The listing builds one solid part. Answer for the finished solid, in the listing's coordinates (mm). A direction names the side the tool comes from. Round coordinates to 2 decimals unless told otherwise and drop trailing zeros. Write each loop counter-clockwise with the first axis right and the second up, starting at its lowest first coordinate (ties: lowest second). Pieces come first, ordered by that corner, then holes.
Item 1: Find the intervals of material crossed by probe 1 along X at (y, z) = (14.55, 10); probe 2 along Z at (x, y) = (14.5, 7); probe 3 along Y at (x, z) = (18, 0), in increasing order.
Item 2: Find section D-D on z = -10.5. Give the vertices of the cut face in (x, y), then the cut area to 3 significant figures.
Item 3: Each of these flat-tipped pins is pushed along its axis until it touches: pin 1 (3 mm diameter, centred on x = -9.5, z = 11, fed in from +Y); pin 2 (5 mm diameter, centred on x = -1, z = 25, fed in from +Y); pin 3 (5 mm diameter, centred on x = 12.5, y = 17.5, fed in from +Z); pin 4 (12 mm diameter, centred on x = 3.5, y = 31.5, fed in from +Z). Where does it stop, or does it pass through?
Item 4: Find section B-B on y = 48. Give the vertices of the cut face in (x, z).
Item 5: Find section C-C on z = -25. Give the vertices of the cut face in (x, y), then the cut area to 3 significant figures.
Item 6: A tool of negligible diameter and unlimited length cuts with its end or side. For faces 5 (the face through (-4.22, 19.4, -21.43)), 6 (the face through (0, 5, -23)), 7 (the face through (-4.22, 19.4, 21.43)), 8 (the face through (16.5, 2.5, 25)), 9 (the face through (-7.97, 18.52, -12.21)), from which of +Z, -Z, +X, -X, +Y, -Y can it reach the whole face along a straight path? Write none if from no direction.
Item 7: For a pull along Z with two mould halves and no side action, classify faces 1 (the face through (-11.464, 14.535, -9.239)), 2 (the face through (0, 3, -23.5)), 3 (the face through (12, 39, 0)), 4 (the face through (0, 4, -35)) as +Z half, -Z half, draft (parallel to the pull), parting line (faces both ways), or undercut.
Item 8: Find section A-A on x = 3. Give the vertices of the cut face in (y, z), then the cut area to 3 significant figures.
```python
from build123d import *

# Parameters (mm, degrees)
SKETCH1_W           = 40
SKETCH1_H           = 70
BOSS_EXTRUDE1_DEPTH = 20
SKETCH2_W           = 30
SKETCH2_H           = 24
CUT_EXTRUDE1_DEPTH  = 57.789083458
SKETCH3_R           = 1.65
CUT_EXTRUDE2_DEPTH  = 46
SKETCH5_R           = 3
CUT_EXTRUDE3_DEPTH  = 3
SKETCH9_W           = 6
SKETCH9_H           = 30
CUT_EXTRUDE6_DEPTH  = 57.789083458
CUT_EXTRUDE7_DEPTH  = 10
SKETCH14_W          = 8
SKETCH14_H          = 44
BOSS_EXTRUDE3_DEPTH = 53
SKETCH16_R          = 6.65
CUT_EXTRUDE11_DEPTH = 88.051708771
SKETCH17_R          = 7.65
CUT_EXTRUDE12_DEPTH = 2
FILLET2_R           = 5
SKETCH18_R          = 3
CUT_EXTRUDE13_DEPTH = 18
CHAMFER1_SIZE       = 2
SKETCH19_W          = 7
SKETCH19_H          = 12
CUT_EXTRUDE14_DEPTH = 91.29950166
FILLET4_R           = 2


with BuildPart() as part:
    # Sketch1 → Boss-Extrude1 (new body)
    with BuildSketch(Plane(origin=(0, 0, 0), x_dir=(1, 0, 0), z_dir=(0, 1, 0))):
        Rectangle(SKETCH1_W, SKETCH1_H)
    extrude(amount=BOSS_EXTRUDE1_DEPTH)

    # Sketch2 → Cut-Extrude1 (cut, through all)
    with BuildSketch(Plane.ZY.offset(20)):
        Rectangle(SKETCH2_W, SKETCH2_H)
    extrude(amount=-CUT_EXTRUDE1_DEPTH, mode=Mode.SUBTRACT)

    # Sketch3 → Cut-Extrude2 (cut, through all)
    with BuildSketch(Plane(origin=(0, 20, 0), x_dir=(1, 0, 0), z_dir=(0, 1, 0))):
        with Locations(Location((-10, 10, 0), (0, 0, 270))):
            Circle(SKETCH3_R)
        with Locations(Location((10, 10, 0), (0, 0, 270))):
            Circle(SKETCH3_R)
        with Locations(Location((10, -10, 0), (0, 0, 270))):
            Circle(SKETCH3_R)
        with Locations(Location((-10, -10, 0), (0, 0, 270))):
            Circle(SKETCH3_R)
    extrude(amount=-CUT_EXTRUDE2_DEPTH, mode=Mode.SUBTRACT)

    # Sketch5 → Cut-Extrude3 (cut)
    with BuildSketch(Plane(origin=(0, 20, 0), x_dir=(1, 0, 0), z_dir=(0, 1, 0))):
        with Locations(Location((-10, 10, 0), (0, 0, 270))):
            Circle(SKETCH5_R)
        with Locations(Location((10, 10, 0), (0, 0, 270))):
            Circle(SKETCH5_R)
        with Locations(Location((10, -10, 0), (0, 0, 270))):
            Circle(SKETCH5_R)
        with Locations(Location((-10, -10, 0), (0, 0, 270))):
            Circle(SKETCH5_R)
    extrude(amount=-CUT_EXTRUDE3_DEPTH, mode=Mode.SUBTRACT)

    # Sketch9 → Cut-Extrude6 (cut, through all)
    with BuildSketch(Plane(origin=(20, 0, 0), x_dir=(0, 0, -1), z_dir=(1, 0, 0))):
        with Locations((25, 20)):
            Rectangle(SKETCH9_W, SKETCH9_H)
    cut_extrude6 = extrude(amount=-CUT_EXTRUDE6_DEPTH, mode=Mode.SUBTRACT)

    # Sketch10 → Cut-Extrude7 (cut)
    with BuildSketch(Plane(origin=(0, 5, 0), x_dir=(1, 0, 0), z_dir=(0, 1, 0))):
        with BuildLine():
            Line((15, 23.5), (-15, 23.5))
            ThreePointArc((-15, 23.5), (-16.5, 25), (-15, 26.5))
            Line((-15, 26.5), (15, 26.5))
            ThreePointArc((15, 26.5), (16.5, 25), (15, 23.5))
        make_face()
    cut_extrude7 = extrude(amount=-CUT_EXTRUDE7_DEPTH, mode=Mode.SUBTRACT)

    # Mirror2: Cut-Extrude6, Cut-Extrude7 across plane
    add(cut_extrude6.mirror(Plane.XY), mode=Mode.SUBTRACT)
    add(cut_extrude7.mirror(Plane.XY), mode=Mode.SUBTRACT)

    # Sketch14 → Boss-Extrude3 (add)
    with BuildSketch(Plane(origin=(0, 20, 0), x_dir=(1, 0, 0), z_dir=(0, 1, 0))):
        with Locations((16, 0)):
            Rectangle(SKETCH14_W, SKETCH14_H)
    extrude(amount=BOSS_EXTRUDE3_DEPTH)

    # Sketch16 → Cut-Extrude11 (cut, through all)
    with BuildSketch(Plane.ZY.offset(-12)):
        with Locations((0, 48)):
            Circle(SKETCH16_R)
    extrude(amount=-CUT_EXTRUDE11_DEPTH, mode=Mode.SUBTRACT)

    # Sketch17 → Cut-Extrude12 (cut)
    with BuildSketch(Plane.ZY.offset(-12)):
        with Locations((0, 48)):
            Circle(SKETCH17_R)
    extrude(amount=-CUT_EXTRUDE12_DEPTH, mode=Mode.SUBTRACT)

    # Fillet2
    fillet2_edges = [part.edges().sort_by_distance(p)[0] for p in [
        (16, 73, -22),
        (16, 73, 22),
    ]]
    fillet(fillet2_edges, radius=FILLET2_R)

    # Sketch18 → Cut-Extrude13 (cut)
    with BuildSketch(Plane(origin=(0, 38, 0), x_dir=(1, 0, 0), z_dir=(0, 1, 0))):
        with Locations(Location((10, 10, 0), (0, 0, 270))):
            Circle(SKETCH18_R)
        with Locations(Location((10, -10, 0), (0, 0, 270))):
            Circle(SKETCH18_R)
    extrude(amount=-CUT_EXTRUDE13_DEPTH, mode=Mode.SUBTRACT)

    # Chamfer1
    # the kernel refuses this chamfer: 2 mm, written as the material it takes off along each edge
    with BuildSketch(Plane(origin=(12, 38, 17.379433953), x_dir=(-0.02749587661058651, 0.9996219169112968, 0), z_dir=(0, 0, -1))) as chamfer1_piece_1_section:
        Polygon((CHAMFER1_SIZE * 0.999621916911, CHAMFER1_SIZE * 0.0274958766106), (-CHAMFER1_SIZE * 0.0274958766106, CHAMFER1_SIZE * 0.999621916911), (0, 0), align=None)
    chamfer1_piece_1 = extrude(amount=14.758867907, mode=Mode.PRIVATE)
    chamfer1_piece_1 = chamfer1_piece_1 & Plane(origin=(10, 38.83392746, 10), x_dir=(0, 0, 1), z_dir=(0, 1, 0)) * Cylinder(3, 38, mode=Mode.PRIVATE)
    add(chamfer1_piece_1, mode=Mode.SUBTRACT)
    with BuildSketch(Plane(origin=(12, 38, -2.620566047), x_dir=(-0.02749587661058651, 0.9996219169112968, 0), z_dir=(0, 0, -1))) as chamfer1_piece_2_section:
        Polygon((CHAMFER1_SIZE * 0.999621916911, CHAMFER1_SIZE * 0.0274958766106), (-CHAMFER1_SIZE * 0.0274958766106, CHAMFER1_SIZE * 0.999621916911), (0, 0), align=None)
    chamfer1_piece_2 = extrude(amount=14.758867907, mode=Mode.PRIVATE)
    chamfer1_piece_2 = chamfer1_piece_2 & Plane(origin=(10, 38.833927472, -10), x_dir=(0, 0, 1), z_dir=(0, 1, 0)) * Cylinder(3, 38, mode=Mode.PRIVATE)
    add(chamfer1_piece_2, mode=Mode.SUBTRACT)

    # Sketch19 → Cut-Extrude14 (cut, through all)
    with BuildSketch(Plane(origin=(20, 0, 0), x_dir=(0, 0, -1), z_dir=(1, 0, 0))):
        with Locations((-31.5, 14)):
            Rectangle(SKETCH19_W, SKETCH19_H)
    cut_extrude14 = extrude(amount=-CUT_EXTRUDE14_DEPTH, mode=Mode.SUBTRACT)

    # Mirror3: Cut-Extrude14 across plane
    add(cut_extrude14.mirror(Plane.XY), mode=Mode.SUBTRACT)

    # Fillet4
    fillet4_edges = [part.edges().sort_by_distance(p)[0] for p in [
        (-4, 20, 22),
        (-4, 20, -22),
    ]]
    fillet(fillet4_edges, radius=FILLET4_R)


solid = part.part
```
Check values:
1. probe 1: x = -20 to -11.65, -8.35 to 8.35, 11.65 to 20
1. probe 2: z = -35 to -28, -22 to -15, 15 to 22, 28 to 35
1. probe 3: y = 12 to 41.35, 54.65 to 73
2. outline: (-20, 12) - (-11.57, 12) - (-11.57, 17) - (-12.96, 17) - (-12.96, 20) - (-20, 20) - close; (-8.43, 12) - (8.43, 12) - (8.43, 17) - (7.04, 17) - (7.04, 20) - (-7.04, 20) - (-7.04, 17) - (-8.43, 17) - close; (11.57, 12) - (20, 12) - (20, 73) - (12, 73) - (12, 40) - (12.96, 39.04) - (12.96, 17) - (11.57, 17) - close
2. area: 658 mm2
3. pin 1: stops at y = 17
3. pin 2: stops at y = 5
3. pin 3: stops at z = 22
3. pin 4: passes through
4. outline: (12, -22) - (20, -22) - (20, -6.65) - (14, -6.65) - (14, -7.65) - (12, -7.65) - close; (12, 7.65) - (14, 7.65) - (14, 6.65) - (20, 6.65) - (20, 22) - (12, 22) - close
5. outline: (-20, 0) - (-16.5, 0) - (-16.5, 5) - (-20, 5) - close; (16.5, 0) - (20, 0) - (20, 5) - (16.5, 5) - close
5. area: 35.0 mm2
6. face 5: -Z, -X, +Y
6. face 6: +X, -X, +Y
6. face 7: +Z, -X, +Y
6. face 8: +Y, -Y
6. face 9: +Y
7. face 1: undercut
7. face 2: undercut
7. face 3: draft
7. face 4: -Z half
8. outline: (0, -35) - (8, -35) - (8, -28) - (5, -28) - (5, -26.5) - (0, -26.5) - close; (0, -23.5) - (5, -23.5) - (5, -22) - (18, -22) arc R2 ccw to (20, -20) - (20, 20) arc R2 ccw to (18, 22) - (5, 22) - (5, 23.5) - (0, 23.5) - (0, 15) - (12, 15) - (12, -15) - (0, -15) - close; (0, 26.5) - (5, 26.5) - (5, 28) - (8, 28) - (8, 35) - (0, 35) - close
8. area: 660 mm2
